```python
from build123d import *

# Parameters (mm, degrees)
SKETCH1_W           = 18.92
SKETCH1_H           = 12.57
BOSS_EXTRUDE1_DEPTH = 0.76
SKETCH2_R           = 0.5
BOSS_EXTRUDE2_DEPTH = 3.55
SKETCH3_W           = 6.416319516
SKETCH3_H           = 5.020284278
BOSS_EXTRUDE3_DEPTH = 5


with BuildPart() as part:
    # Sketch1 → Boss-Extrude1 (new body)
    with BuildSketch(Plane(origin=(0, 0, 0), x_dir=(1, 0, 0), z_dir=(0, 1, 0))):
        with Locations((9.46, -6.285)):
            Rectangle(SKETCH1_W, SKETCH1_H)
    extrude(amount=BOSS_EXTRUDE1_DEPTH)

    # Sketch2 → Boss-Extrude2 (add)
    with BuildSketch(Plane(origin=(0, 0, 0), x_dir=(-1, 0, 0), z_dir=(0, -1, 0))):
        with Locations(Location((-2.02, -11.07, 0), (0, 0, 270))):
            Circle(SKETCH2_R)
        with Locations(Location((-17.9, -11.07, 0), (0, 0, 270))):
            Circle(SKETCH2_R)
        with Locations(Location((-2.02, -7.89, 0), (0, 0, 270))):
            Circle(SKETCH2_R)
        with Locations(Location((-2.02, -1.54, 0), (0, 0, 270))):
            Circle(SKETCH2_R)
        with Locations(Location((-17.9, -1.54, 0), (0, 0, 270))):
            Circle(SKETCH2_R)
    extrude(amount=BOSS_EXTRUDE2_DEPTH)

    # Sketch3 → Boss-Extrude3 (add)
    with BuildSketch(Plane(origin=(0, 0.76, 0), x_dir=(1, 0, 0), z_dir=(0, 1, 0))):
        with Locations((14.691840242, -6.022310706)):
            Rectangle(SKETCH3_W, SKETCH3_H)
    extrude(amount=BOSS_EXTRUDE3_DEPTH)


solid = part.part
```
Geometry: final body of the model. Coordinates: model frame, mm. A direction names the side the tool comes from. Coordinates: 2 decimals unless noted, no trailing zeros. Loops run counter-clockwise (first coordinate to the right, second up) from the corner with the lowest first, then second, coordinate; pieces in that order, holes last. Notation, with made-up numbers: M -17,-7 L -10,-7 A32 ccw -10,23 Z; hole C 87,34.25 d11. An arc over 180 degrees is marked long. Put each result on its own line as item: value.
(1) Cut plane B-B on x = 12.25. Return the cut outline in (y, z).
Answer sheet:
outline: M 0,0 L 0.76,0 L 0.76,3.51 L 5.76,3.51 L 5.76,8.53 L 0.76,8.53 L 0.76,12.57 L 0,12.57 Z
(2) First-contact query: pin 1 (1 mm diameter, centred on y = 3, z = 10, fed in from +X); pin 2 (3 mm diameter, centred on x = 4, z = 10, fed in from +Y); pin 3 (1.5 mm diameter, centred on y = -2, z = 1.5, fed in from -X); pin 4 (4 mm diameter, centred on x = 7.5, z = 6.5, fed in from -Y). Flat tips, straight axial feed; report the tip coordinate or a pass-through.
Answer sheet:
pin 1: passes through
pin 2: stops at y = 0.76
pin 3: stops at x = 1.52
pin 4: stops at y = 0
(3) Draft query along X for faces 1 (the face through (15, 3, 8.532)), 2 (the face through (2.212, -1.75, 11.532)), 3 (the face through (2.32, -1.75, 7.49)), 4 (the face through (11.484, 3, 6)). Return one class per face: pulls with the +X half, pulls with the -X half, needs draft (parallel to the pull), parting line crosses it, or undercut.
Answer sheet:
face 1: needs draft
face 2: undercut
face 3: parting line crosses it
face 4: pulls with the -X half
(4) Cut plane D-D on z = 7.89. Return the cut outline in (x, y), then the cut area to 3 significant figures.
Answer sheet:
outline: M 0,0 L 1.52,0 L 1.52,-3.55 L 2.52,-3.55 L 2.52,0 L 18.92,0 L 18.92,0.76 L 17.9,0.76 L 17.9,5.76 L 11.48,5.76 L 11.48,0.76 L 0,0.76 Z
area: 50.0 mm^2
(5) Material intervals for probe 1 along X at (y, z) = (2.75, 4); probe 2 along Y at (x, z) = (17.25, 4.75); probe 3 along Y at (x, z) = (13.5, 9), sorted ascending.
Answer sheet:
probe 1: x = 11.48 to 17.9
probe 2: y = 0 to 5.76
probe 3: y = 0 to 0.76
(6) Cut plane C-C on y = 3. Return the cut outline in (x, z).
Answer sheet:
outline: M 11.48,3.51 L 17.9,3.51 L 17.9,8.53 L 11.48,8.53 Z
(7) Cut plane A-A on z = 1.54. Return the cut outline in (x, y), then the cut area to 3 significant figures.
Answer sheet:
outline: M 0,0 L 1.52,0 L 1.52,-3.55 L 2.52,-3.55 L 2.52,0 L 17.4,0 L 17.4,-3.55 L 18.4,-3.55 L 18.4,0 L 18.92,0 L 18.92,0.76 L 0,0.76 Z
area: 21.5 mm^2
(8) Access query for faces 5 (the face through (17.9, 3, 6)), 6 (the face through (2.5, -1.8, 1.4)), 7 (the face through (15, 3, 3.512)). Directions: +Z, -Z, +X, -X, +Y, -Y. A direction counts if a zero-diameter tool reaches every point of the face in a straight line with its end or side. Return the directions, or none.
Answer sheet:
face 5: +Z, -Z, +X, +Y
face 6: -Y
face 7: -Z, +X, -X, +Y
